Check sheet for the modelled part. Datum: model origin and axes. Units: mm. A direction names the side the tool comes from. Give positions to 0.01 mm unless a question says otherwise; leave off trailing zeros. Write each loop counter-clockwise with the first axis right and the second up, starting at its lowest first coordinate (ties: lowest second). Pieces come first, ordered by that corner, then holes. Notation, with made-up numbers: (72, 44.5) -> (86, 44.5) arc R11 cw to (86, 51.5) -> close; hole circle Ø3 at (42.25, 80). An arc over 180 degrees is marked (long way). Use a Markdown table: item, result. Add a question column.
1. Gauge pin test, flat ends, axial feed: P1, Ø1, axis at y = -28.5, z = 3.5, coming from the +X side; P2, Ø5, axis at y = -34, z = 1, coming from the -X side; P3, Ø3, axis at y = -14.5, z = 5, coming from the +X side. Record the tip position at first contact, or that the pin passes through.
2. Cross-section at B-B (z = 2). Enter the section's corners in (x, y).
3. Cross-section at A-A (x = -7.25). Enter the section's corners in (y, z).
4. Cross-section at C-C (y = -58.5). Enter the section's corners in (x, z).
5. Set-up check for faces 4 (the flat face through (-5.303, -56.923, 4.93)), 5 (the cylindrical face through (-1.163, -80.599, 4.93)): record each of +Z, -Z, +X, -X, +Y, -Y from which the full face is reachable in a straight line by a thin tool's end or side.
6. Cross-section at D-D (x = -13.25). Enter the section's corners in (y, z).
7. Scan lines: probe 1 along X at (y, z) = (-38, 4.5); probe 2 along X at (y, z) = (-26, 4.5). Record each from-to range of solid material in increasing order. Write a range as [from, to].
8. Release check for a two-part mould opening along Y. For faces 1 (the flat face through (-4.93, -19.09, 4.93)), 2 (the flat face through (-10, -43, 10)), 3 (the flat face through (-1.909, 0.493, 4.93)) record: released by +Y, released by -Y, zero draft, split by the parting line, or undercut.
Autodesk Inventor part; units mm, degrees
ref_plane "YZ Plane" through (0, 0, 0) normal (1, 0, 0) x (0, 1, 0)
ref_plane "XZ Plane" through (0, 0, 0) normal (0, 1, 0) x (-1, 0, 0)
ref_plane "XY Plane" through (0, 0, 0) normal (0, 0, 1) x (1, 0, 0)
sketch "Sketch1 - gripper" plane through (0, 0, 0) normal (0, 0, 1) x (1, 0, 0)
  line L0 (0, 0) -> (-10, -38.7298)
  line L1 (-10, -38.7298) -> (0, -38.7298) construction
  line L2 (-10, -38.7298) -> (0, -77.4597)
  line L3 (0, 0) -> (-3.873, 1)
  line L4 (-3.873, 1) -> (-14.3579, -37.8519)
  line L5 (-14.3579, -37.8519) -> (-3.873, -78.4597)
  line L6 (-3.873, -78.4597) -> (0, -77.4597)
  circle A0 centre (-1.9365, -77.9597) radius 2.75
  point P0 (-4.3448, -76.6321)
  point P1 (-0.4719, -75.6321)
  dimension "d18" = 40
  dimension "d19" = 40
  dimension "d20" = 4
  dimension "d21" = 5.5
extrude "Extrusion1" add sketch "Sketch1 - gripper" along normal blind 10
sketch "Sketch3" plane through (0, 0, 0) normal (0, 0, -1) x (-1, 0, 0)
  line L0 (10, -38.7298) -> (0, 0) construction
  line L1 (3.873, 1) -> (14.3579, -37.8519)
  line L2 (4.1429, 0) -> (-40.8571, 0)
  line L3 (-40.8571, 0) -> (-40.8571, 25)
  line L4 (-40.8571, 25) -> (4.1429, 25)
  line L5 (4.1429, 25) -> (4.1429, 0)
  dimension "d22" = 45
  dimension "d23" = 25
properties part number "arm1"
Worked answers:
| question | item | result |
|---|---|---|
| 1 | P1 | stops at x = -7.23 |
| 1 | P2 | stops at x = -13.99 |
| 1 | P3 | stops at x = -3.36 |
| 2 | outline | (-14.36, -37.85) -> (-4.34, -76.63) arc R2.75 ccw (long way) to (-0.47, -75.63) -> (-10, -38.73) -> (0, 0) -> (-3.87, 1) -> close |
| 3 | outline | (-65.38, 0) -> (-49.38, 0) -> (-49.38, 10) -> (-65.38, 10) -> close; (-28.08, 0) -> (-11.51, 0) -> (-11.51, 10) -> (-28.08, 10) -> close |
| 4 | outline | (-9.03, 0) -> (-4.9, 0) -> (-4.9, 10) -> (-9.03, 10) -> close |
| 5 | face 4 | +Z, -Z, +X |
| 5 | face 5 | +Z, -Z |
| 6 | outline | (-42.14, 0) -> (-33.75, 0) -> (-33.75, 10) -> (-42.14, 10) -> close |
| 7 | probe 1 | x = [-14.32, -9.81] |
| 7 | probe 2 | x = [-11.16, -6.71] |
| 8 | face 1 | undercut |
| 8 | face 2 | zero draft |
| 8 | face 3 | released by +Y |
